```python
from build123d import *

# Parameters (mm, degrees)
BOSS_EXTRUDE1_DEPTH     = 12.7
CUT_EXTRUDE2_DEPTH      = 52.709076543
CUT_EXTRUDE2_DEPTH_BACK = 12.7
SKETCH4_W               = 5.555555556
SKETCH4_H               = 5.954243766
BOSS_EXTRUDE2_DEPTH     = 7


with BuildPart() as part:
    # Sketch2 → Boss-Extrude1 (new body)
    with BuildSketch(Plane(origin=(0, 0, 0), x_dir=(1, 0, 0), z_dir=(0, 1, 0))):
        with BuildLine():
            Line((36.805555556, 34.027777778), (36.805555556, 28.472222222))
            Line((36.805555556, 28.472222222), (28.059895833, 28.472222222))
            Line((28.059895833, 28.472222222), (27.311197917, 17.274305556))
            add(Edge.make_bspline(
                [(27.311197917, 17.274305556), (27.277795656, 16.804166639), (27.213581874, 15.900353642), (27.134284285, 14.591279231), (27.088344823, 13.379251723), (27.084956214, 12.601307574), (27.083333333, 12.228732639)],
                knots=[0, 0, 0, 0, 1.119532368, 2.152231754, 3.115062263, 4, 4, 4, 4], degree=3))
            add(Edge.make_bspline(
                [(27.083333333, 12.228732639), (27.088274581, 11.823604319), (27.097676522, 11.052747972), (27.1463749, 9.958919939), (27.245170271, 8.988755862), (27.371002693, 8.143926135), (27.529152233, 7.419430528), (27.728457334, 6.818301639), (27.97650636, 6.339464464), (28.352227221, 5.878445418), (28.902546694, 5.47047021), (29.612022333, 5.12581616), (30.381545964, 4.888099058), (30.919027092, 4.870283408), (31.195746528, 4.861111111)],
                knots=[0, 0, 0, 0, 1.508120221, 2.869569927, 4.073906796, 5.136392291, 6.047624064, 6.831039609, 7.487569696, 8.042672177, 9.031004047, 10.006413578, 10.97361213, 12, 12, 12, 12], degree=3))
            add(Edge.make_bspline(
                [(31.195746528, 4.861111111), (31.47916585, 4.872136088), (32.020929674, 4.893210634), (32.788220791, 5.094099051), (33.466107529, 5.423211567), (34.05259416, 5.891325855), (34.548953998, 6.488400226), (34.936220725, 7.22238631), (35.244986398, 8.076473761), (35.357486114, 8.699850181), (35.416666667, 9.027777778)],
                knots=[0, 0, 0, 0, 1.033647866, 1.975846305, 2.874029418, 3.767535477, 4.696297243, 5.689637366, 6.784632136, 8, 8, 8, 8], degree=3))
            Line((35.416666667, 9.027777778), (36.805555556, 9.027777778))
            add(Edge.make_bspline(
                [(36.805555556, 9.027777778), (36.751313392, 8.636593642), (36.645430641, 7.872987448), (36.430993277, 6.771079076), (36.1666915, 5.743505172), (35.873825885, 4.788096172), (35.503638642, 3.918308722), (35.126438428, 3.108890157), (34.67022236, 2.39005292), (34.190460036, 1.734735752), (33.64770155, 1.167708505), (33.078282467, 0.661363985), (32.447526517, 0.251271838), (31.785619175, -0.107880779), (31.064059185, -0.356214557), (30.308826122, -0.563500536), (29.502063403, -0.664205141), (28.949843487, -0.684214933), (28.667534722, -0.694444444)],
                knots=[0, 0, 0, 0, 1.346490984, 2.628401203, 3.824883511, 4.963792231, 6.031069444, 7.045970716, 8.004214277, 8.929182016, 9.810359102, 10.675861826, 11.520733207, 12.370272421, 13.236390006, 14.115839292, 15.03676947, 16, 16, 16, 16], degree=3))
            add(Edge.make_bspline(
                [(28.667534722, -0.694444444), (28.154682861, -0.675816782), (27.164131243, -0.639838242), (25.766335044, -0.242024901), (24.512145619, 0.369174112), (23.621609051, 1.101026149), (23.010255911, 1.797210882), (22.609852371, 2.383817061), (22.268478936, 3.030858971), (22.003101082, 3.740487332), (21.782965902, 4.501315843), (21.632459475, 5.322642072), (21.547875637, 6.204798769), (21.53462541, 6.814049436), (21.527777778, 7.12890625)],
                knots=[0, 0, 0, 0, 1.53176672, 2.958542455, 4.314758716, 5.68491526, 6.375705814, 7.084681483, 7.806528549, 8.560798466, 9.349284224, 10.175616502, 11.057170379, 12, 12, 12, 12], degree=3))
            add(Edge.make_bspline(
                [(21.527777778, 7.12890625), (21.530511411, 7.37125412), (21.536674087, 7.917600965), (21.569321673, 8.825873224), (21.639359606, 9.910585643), (21.725996598, 11.172904628), (21.834635018, 12.612456183), (21.96658957, 14.232690848), (22.114735136, 16.030968586), (22.235168036, 17.288909187), (22.298177083, 17.947048611)],
                knots=[0, 0, 0, 0, 0.536190643, 1.208783333, 2.010417809, 2.94084931, 4.00811323, 5.204264869, 6.537304937, 8, 8, 8, 8], degree=3))
            Line((22.298177083, 17.947048611), (23.285590278, 28.472222222))
            Line((23.285590278, 28.472222222), (15.277777778, 28.472222222))
            add(Edge.make_bspline(
                [(15.277777778, 28.472222222), (15.214460278, 27.401507925), (15.092072877, 25.331907254), (14.886109564, 22.340596723), (14.670777515, 19.573381685), (14.442846588, 17.030553937), (14.208342944, 14.71137929), (13.954506302, 12.617981517), (13.715610292, 10.74508508), (13.436521107, 9.086740026), (13.164846669, 7.602952782), (12.886850841, 6.270387957), (12.590238795, 5.07441313), (12.303899426, 4.011159992), (12.003972777, 3.085637953), (11.686744628, 2.301603715), (11.378814424, 1.642404725), (10.958043065, 0.964152103), (10.358101863, 0.292051075), (9.505081424, -0.285187523), (8.526340218, -0.641645855), (7.833640049, -0.676470824), (7.476128472, -0.694444444)],
                knots=[0, 0, 0, 0, 2.01044623, 3.886023449, 5.620111306, 7.212895615, 8.671360263, 9.989066837, 11.16552434, 12.209857215, 13.140654073, 13.99296191, 14.760845937, 15.449993852, 16.056713946, 16.582946555, 17.034739681, 17.418487115, 18.076100987, 18.706013306, 19.33215662, 20, 20, 20, 20], degree=3))
            add(Edge.make_bspline(
                [(7.476128472, -0.694444444), (7.207412809, -0.681627697), (6.681489385, -0.656543087), (5.927311086, -0.469815134), (5.234803565, -0.159026243), (4.623769653, 0.271526397), (4.10585267, 0.797998542), (3.737602188, 1.427988796), (3.515453468, 2.133829731), (3.486861324, 2.631486012), (3.472222222, 2.886284722)],
                knots=[0, 0, 0, 0, 1.073515936, 2.101057932, 3.084730514, 4.091615775, 5.073373561, 6.013242394, 6.982785322, 8, 8, 8, 8], degree=3))
            add(Edge.make_bspline(
                [(3.472222222, 2.886284722), (3.49977796, 3.167601475), (3.56174898, 3.800264126), (3.975195909, 4.785596558), (4.58793497, 5.912424554), (5.130000946, 6.671771181), (5.425347222, 7.085503472)],
                knots=[0, 0, 0, 0, 0.719350384, 1.617771125, 2.702035439, 4, 4, 4, 4], degree=3))
            add(Edge.make_bspline(
                [(5.425347222, 7.085503472), (5.880890291, 7.733268934), (6.778468477, 9.009592048), (7.924062056, 11.019134082), (8.912809694, 13.051591024), (9.583491505, 14.814505434), (10.052627408, 16.316401679), (10.355193153, 17.603017915), (10.666713374, 19.033013262), (10.926646603, 20.624922957), (11.194761694, 22.366552488), (11.410609585, 24.268277428), (11.637107009, 26.317618199), (11.748122743, 27.737606389), (11.805555556, 28.472222222)],
                knots=[0, 0, 0, 0, 1.256859471, 2.476450027, 3.668368903, 4.842737386, 5.467680022, 6.165560467, 6.940549266, 7.791280764, 8.726175375, 9.738470097, 10.830021485, 12, 12, 12, 12], degree=3))
            Line((11.805555556, 28.472222222), (9.407552083, 28.472222222))
            add(Edge.make_bspline(
                [(9.407552083, 28.472222222), (8.954085196, 28.460620671), (8.094301289, 28.438623856), (6.890732805, 28.196638527), (5.842130851, 27.81794011), (4.969568852, 27.229936528), (4.197964836, 26.514921386), (3.47646424, 25.663099106), (2.739413588, 24.704465568), (2.307624449, 23.984891132), (2.083333333, 23.611111111)],
                knots=[0, 0, 0, 0, 1.164670171, 2.208242094, 3.144640406, 4.011598175, 4.893941805, 5.843464191, 6.879796223, 8, 8, 8, 8], degree=3))
            Line((2.083333333, 23.611111111), (0.694444444, 23.611111111))
            add(Edge.make_bspline(
                [(0.694444444, 23.611111111), (0.877085401, 24.232597394), (1.229291, 25.431074191), (1.886266978, 27.119888333), (2.60411942, 28.642568556), (3.40397479, 29.980706486), (4.259111756, 31.115981615), (5.118517845, 32.058955597), (5.996672541, 32.785861584), (6.772590288, 33.224850634), (7.449074281, 33.455523285), (8.027104125, 33.619326955), (8.696031334, 33.743397524), (9.444623844, 33.855790163), (10.28602055, 33.921881494), (11.211287579, 33.993942488), (12.22496831, 34.020966417), (12.926797761, 34.025446099), (13.292100694, 34.027777778)],
                knots=[0, 0, 0, 0, 1.702237036, 3.282601159, 4.758360036, 6.123233304, 7.372634412, 8.489452943, 9.469553166, 10.358928799, 10.813046741, 11.345939706, 11.937066667, 12.599998432, 13.335161994, 14.154869419, 15.039607681, 16, 16, 16, 16], degree=3))
            Line((13.292100694, 34.027777778), (36.805555556, 34.027777778))
        make_face()
    extrude(amount=BOSS_EXTRUDE1_DEPTH)

    # Sketch3 → Cut-Extrude2 (cut, two sides: drawn at the far end of the back side and taken through both)
    with BuildSketch(Plane(origin=(0, 12.7, 0), x_dir=(1, 0, 0), z_dir=(0, 1, 0)).offset(-CUT_EXTRUDE2_DEPTH_BACK)):
        with BuildLine():
            Line((15.277777778, 28.472222222), (11.805555556, 28.472222222))
            add(Edge.make_bspline(
                [(11.805555556, 28.472222222), (11.748122743, 27.737606389), (11.637107009, 26.317618199), (11.410609585, 24.268277428), (11.194761694, 22.366552488), (10.926646603, 20.624922957), (10.666713374, 19.033013262), (10.355193153, 17.603017915), (10.052627408, 16.316401679), (9.583491505, 14.814505434), (8.912809694, 13.051591024), (7.924062056, 11.019134082), (6.778468477, 9.009592048), (5.880890291, 7.733268934), (5.425347222, 7.085503472)],
                knots=[0, 0, 0, 0, 0.09749821, 0.188460825, 0.272818719, 0.350726603, 0.421620894, 0.486203294, 0.544359998, 0.596438551, 0.694302591, 0.793629164, 0.895261711, 1, 1, 1, 1], degree=3))
            add(Edge.make_bspline(
                [(5.425347222, 7.085503472), (5.130000946, 6.671771181), (4.58793497, 5.912424554), (3.975195909, 4.785596558), (3.56174898, 3.800264126), (3.49977796, 3.167601475), (3.472222222, 2.886284722)],
                knots=[0, 0, 0, 0, 0.32449114, 0.595557219, 0.820162404, 1, 1, 1, 1], degree=3))
            add(Edge.make_bspline(
                [(3.472222222, 2.886284722), (3.486861324, 2.631486012), (3.515453468, 2.133829731), (3.737602188, 1.427988796), (4.10585267, 0.797998542), (4.623769653, 0.271526397), (5.234803565, -0.159026243), (5.927311086, -0.469815134), (6.681489385, -0.656543087), (7.207412809, -0.681627697), (7.476128472, -0.694444444)],
                knots=[0, 0, 0, 0, 0.127151835, 0.248344701, 0.365828305, 0.488548028, 0.614408686, 0.737367758, 0.865810508, 1, 1, 1, 1], degree=3))
            add(Edge.make_bspline(
                [(7.476128472, -0.694444444), (7.833640049, -0.676470824), (8.526340218, -0.641645855), (9.505081424, -0.285187523), (10.358101863, 0.292051075), (10.958043065, 0.964152103), (11.378814424, 1.642404725), (11.686744628, 2.301603715), (12.003972777, 3.085637953), (12.303899426, 4.011159992), (12.590238795, 5.07441313), (12.886850841, 6.270387957), (13.164846669, 7.602952782), (13.436521107, 9.086740026), (13.715610292, 10.74508508), (13.954506302, 12.617981517), (14.208342944, 14.71137929), (14.442846588, 17.030553937), (14.670777515, 19.573381685), (14.886109564, 22.340596723), (15.092072877, 25.331907254), (15.214460278, 27.401507925), (15.277777778, 28.472222222)],
                knots=[0, 0, 0, 0, 0.033392169, 0.064699335, 0.096194951, 0.129075644, 0.148263016, 0.170852672, 0.197164303, 0.227500307, 0.261957703, 0.300351905, 0.342967296, 0.389507139, 0.441723783, 0.500546658, 0.566431987, 0.639355219, 0.718994435, 0.805698828, 0.899477689, 1, 1, 1, 1], degree=3))
        make_face()
        with BuildLine():
            Line((9.591392396, 33.862133441), (9.591392396, 28.472222222))
            Line((9.591392396, 28.472222222), (11.805555556, 28.472222222))
            Line((11.805555556, 28.472222222), (15.277777778, 28.472222222))
            Line((15.277777778, 28.472222222), (16.237282416, 28.472222222))
            Line((16.237282416, 28.472222222), (16.237282416, 34.027777778))
            Line((16.237282416, 34.027777778), (13.292100694, 34.027777778))
            add(Edge.make_bspline(
                [(13.292100694, 34.027777778), (12.926797761, 34.025446099), (12.22496831, 34.020966417), (11.211287579, 33.993942488), (10.343864349, 33.926386444), (9.811849706, 33.884631797), (9.591392396, 33.862133441)],
                knots=[0, 0, 0, 0, 0.06002452, 0.115320661, 0.166552375, 0.202967967, 0.202967967, 0.202967967, 0.202967967], degree=3))
        make_face()
    extrude(amount=CUT_EXTRUDE2_DEPTH + CUT_EXTRUDE2_DEPTH_BACK, mode=Mode.SUBTRACT)


with BuildPart() as cut_extrude2_piece_1:
    # of the separate pieces the step leaves, piece 1, a body of its own (cut_extrude2_pieces)
    add(part.part.solids().sort_by_distance((36.805555556, 0, -34.027777778))[0])



with BuildPart() as cut_extrude2_piece_2:
    # of the separate pieces the step leaves, piece 2, a body of its own (cut_extrude2_pieces)
    add(part.part.solids().sort_by_distance((0.694444444, 0, -23.611111111))[0])


with BuildPart() as cut_extrude2_piece_1_1:
    add(cut_extrude2_piece_1.part)

    add(cut_extrude2_piece_2.part)  # Boss-Extrude2 merges Cut-Extrude2 piece 2
    # Sketch4 → Boss-Extrude2 (add)
    with BuildSketch(Plane.ZY.offset(-16.237282416)):
        with Locations((-31.25, 2.977121883)):
            Rectangle(SKETCH4_W, SKETCH4_H)
    extrude(amount=BOSS_EXTRUDE2_DEPTH)


solid = cut_extrude2_piece_1_1.part
```
Can you work these out from the model? Positions are in its coordinate system, mm. A direction names the side the tool comes from. Round coordinates to 2 decimals unless told otherwise and drop trailing zeros. Loops run counter-clockwise (first coordinate to the right, second up) from the corner with the lowest first, then second, coordinate; pieces in that order, holes last. Notation, with made-up numbers: M 66,37 L 73,37 A12 ccw 73,54 Z; hole C 86,68 d6. An arc over 180 degrees is marked long. Answer as a JSON object with one key per item and string values. Group by question number.
Q1. Please list where these lines run through material, in increasing order: L1, parallel to Z at x = 18, y = 10; L2, parallel to Z at x = 35, y = 11.75; L3, parallel to Z at x = 30, y = 2.75.
Q2. We'd pull the mould along X, two halves only. Please class faces 5 (the flat face through (36.806, 6, -31)), 6 (the flat face through (32, 6, -28.472)), 7 (the flat face through (22.785, 6.261, -23.136)): +X half, -X half, draft (parallel to the pull), parting line (faces both ways), or undercut.
Q3. Imagine slicing it at A-A, the plane x = 17.5. Please give me the cut outline in (y, z), then the cut area to 3 significant figures.
Q4. On a 3-axis mill with a long thin cutter (end or side, diameter ignored), from which of +Z, -Z, +X, -X, +Y, -Y can I reach the whole of each face in a straight line? I mean faces 1 (the flat face through (1, 6, -23.611)), 2 (the flat face through (18, 5, -28.472)), 3 (the flat face through (27.69, 6.26, -22.95)), 4 (the flat face through (9.591, 9, -31)). Say none if no direction works.
Q5. Will these pins go through, and if not, where does the flat tip stop? pin 1 (1.5 mm diameter, centred on x = 1.5, y = 8, fed in from +Z); pin 2 (5 mm diameter, centred on y = 6, z = -7, fed in from -X); pin 3 (7 mm diameter, centred on x = 34, y = 5, fed in from +Z).
Q6. Imagine slicing it at B-B, the plane z = -22. Please give me the cut outline in (x, y), then the cut area to 3 significant figures.
Findings:
{
 "1": {"L1": "z = -34.03 to -28.47", "L2": "z = -34.03 to -28.47, -7.43 to -2.92", "L3": "z = -34.03 to -28.47, -5.01 to 0.6"},
 "2": {"face 5": "+X half", "face 6": "draft", "face 7": "undercut"},
 "3": {"outline": "M 0,-34.03 L 12.7,-34.03 L 12.7,-28.47 L 0,-28.47 Z", "area": "70.6 mm2"},
 "4": {"face 1": "+Z, -X, +Y, -Y", "face 2": "+Y, -Y", "face 3": "+X, +Y, -Y", "face 4": "+Z, -Z, +Y"},
 "5": {"pin 1": "stops at z = -23.61", "pin 2": "stops at x = 21.53", "pin 3": "stops at z = 0.5"},
 "6": {"outline": "M 22.68,0 L 27.63,0 L 27.63,12.7 L 22.68,12.7 Z", "area": "62.8 mm2"}
}
